Geometry check sheet. Reference: the model listing, model coordinates, mm. A direction names the side the tool comes from. Give positions to 0.01 mm unless a question says otherwise; leave off trailing zeros. Loops run counter-clockwise (first coordinate to the right, second up) from the corner with the lowest first, then second, coordinate; pieces in that order, holes last.
1. Cross-section at D-D, the plane z = 22.5. Record the cut outline in (x, y), plus the area to 3 significant figures.
2. Tool access check on faces 4 (the flat face through (7.5, -0.1, 0.5)), 5 (the cylindrical face through (-0.521, 29.76, 18.534)), 6 (the flat face through (0, -29, 16)). Record the directions out of +Z, -Z, +X, -X, +Y, -Y that give a thin tool (end or side, any length) a straight path to the whole face; none if there is none.
3. Go/stop test with flat-tipped pins: pin 1 Ø10 at (y, z) = (20, 16.5) entering from -X; pin 2 Ø4 at (x, y) = (5, 9.5) entering from +Z; pin 3 Ø4.5 at (x, z) = (-1, 22) entering from +Y. Record where each tip stops, or that it passes through.
4. Release check for a two-part mould opening along Z. For faces 1 (the flat face through (-5, 0, 1.5)), 2 (the cylindrical face through (0, -30, 21)), 3 (the flat face through (0, 29, 16)) record: +Z half, -Z half, draft (parallel to the pull), parting line (faces both ways), or undercut.
5. Cross-section at B-B, the plane x = 0. Record the cut outline in (y, z), plus the area to 3 significant figures.
6. Cross-section at A-A, the plane z = 8.25. Record the cut outline in (x, y), plus the area to 3 significant figures.
7. Material ranges on L1, parallel to X at y = 30.05, z = 22.5; L2, parallel to Z at x = 0, y = 29.4; L3, parallel to Z at x = 0, y = -29.35, recorded low to high.
8. Cross-section at C-C, the plane y = 0. Record the cut outline in (x, z).
from build123d import *

# Parameters (mm, degrees)
SKETCH1_R           = 4
BOSS_EXTRUDE1_DEPTH = 1.5
SKETCH2_W           = 15
SKETCH2_H           = 1.5
BOSS_EXTRUDE2_DEPTH = 28.5
SKETCH3_R           = 1.5
CUT_EXTRUDE1_DEPTH  = 62
FILLET1_R           = 1
CUT_EXTRUDE2_REACH  = 63
SKETCH5_R           = 4


with BuildPart() as part:
    # Sketch1 → Boss-Extrude1 (new body)
    with BuildSketch(Plane.XY):
        Polygon((-7.5, -23.042592662), (-7.5, -30.5), (7.5, -30.5), (7.5, -23.042592662), (7.5, 26.84732779), (7.5, 30.5), (-7.5, 30.5), (-7.5, 26.84732779), align=None)
        Circle(SKETCH1_R, mode=Mode.SUBTRACT)
    extrude(amount=BOSS_EXTRUDE1_DEPTH)

    # Sketch2 → Boss-Extrude2 (add)
    with BuildSketch(Plane.XY.offset(1.5)):
        with Locations((0, 29.75)):
            Rectangle(SKETCH2_W, SKETCH2_H)
        with Locations((0, -29.75)):
            Rectangle(SKETCH2_W, SKETCH2_H)
    extrude(amount=BOSS_EXTRUDE2_DEPTH)

    # Sketch3 → Cut-Extrude1 (cut, through all)
    with BuildSketch(Plane(origin=(0, 30.5, 0), x_dir=(1, 0, 0), z_dir=(0, 1, 0))):
        with Locations((0, -22.5)):
            Circle(SKETCH3_R)
    extrude(amount=-CUT_EXTRUDE1_DEPTH, mode=Mode.SUBTRACT)

    # Fillet1
    fillet1_edges = [part.edges().sort_by_distance(p)[0] for p in [
        (0, -30.5, 0),
        (-7.5, -29.75, 30),
        (7.5, -29.75, 30),
        (7.5, 29.75, 30),
        (-7.5, 29.75, 30),
        (0, 30.5, 0),
    ]]
    fillet(fillet1_edges, radius=FILLET1_R)

    # Sketch5 → Cut-Extrude2 (cut, up to next)
    with BuildSketch(Plane(origin=(0, 30.5, 0), x_dir=(1, 0, 0), z_dir=(0, 1, 0)), mode=Mode.PRIVATE) as cut_extrude2_sk1:
        with Locations((0, -22.5)):
            Circle(SKETCH5_R)
    cut_extrude2_tool1 = extrude(cut_extrude2_sk1.sketch, amount=-CUT_EXTRUDE2_REACH, mode=Mode.PRIVATE) & part.part
    add(cut_extrude2_tool1.solids().sort_by_distance((0, 30.5, 22.5))[0], mode=Mode.SUBTRACT)


solid = part.part
Result:
1. outline: (-7.5, -30.5) - (-1.5, -30.5) - (-1.5, -29) - (-7.5, -29) - close; (-7.5, 29) - (-4, 29) - (-4, 30.5) - (-7.5, 30.5) - close; (1.5, -30.5) - (7.5, -30.5) - (7.5, -29) - (1.5, -29) - close; (4, 29) - (7.5, 29) - (7.5, 30.5) - (4, 30.5) - close
1. area: 28.5 mm2
2. face 4: +Z, -Z, +X, +Y, -Y
2. face 5: +Y
2. face 6: +Z, +X, -X
3. pin 1: passes through
3. pin 2: stops at z = 1.5
3. pin 3: stops at y = -29
4. face 1: +Z half
4. face 2: undercut
4. face 3: draft
5. outline: (-30.5, 1) arc R1 ccw to (-29.5, 0) - (-4, 0) - (-4, 1.5) - (-29, 1.5) - (-29, 21) - (-30.5, 21) - close; (-30.5, 24) - (-29, 24) - (-29, 30) - (-30.5, 30) - close; (4, 0) - (29.5, 0) arc R1 ccw to (30.5, 1) - (30.5, 18.5) - (29, 18.5) - (29, 1.5) - (4, 1.5) - close; (29, 26.5) - (30.5, 26.5) - (30.5, 30) - (29, 30) - close
5. area: 148 mm2
6. outline: (-7.5, -30.5) - (7.5, -30.5) - (7.5, -29) - (-7.5, -29) - close; (-7.5, 29) - (7.5, 29) - (7.5, 30.5) - (-7.5, 30.5) - close
6. area: 45.0 mm2
7. L1: x = -7.5 to -4, 4 to 7.5
7. L2: z = 0 to 18.5, 26.5 to 30
7. L3: z = 0 to 21, 24 to 30
8. outline: (-7.5, 0) - (-4, 0) - (-4, 1.5) - (-7.5, 1.5) - close; (4, 0) - (7.5, 0) - (7.5, 1.5) - (4, 1.5) - close
